Work out the finished part from the listing and answer in its coordinate system (mm). A direction names the side the tool comes from. Round coordinates to 2 decimals unless told otherwise and drop trailing zeros. Order: outer loops, then holes, each group sorted by start corner. A loop starts at its lowest first (then second) coordinate and runs counter-clockwise, first axis right, second up. Notation, with made-up numbers: (26.25, 23) -> (69.25, 23) arc R18 ccw to (69.25, 30) -> close; hole circle Ø8 at (18, -36). An arc over 180 degrees is marked (long way). Use a Markdown table: item, result. Add a question column.
Item 1: A cutting plane is placed at D-D, the plane y = 37. Determine the outline of the cut face in (x, z), plus the area to 3 significant figures.
Item 2: For a pull along X with two mould halves and no side action, classify faces 4 (the flat face through (-15.989, 44.684, -33.256)), 5 (the flat face through (0, 53, -38.354)), 6 (the flat face through (16.079, 99.775, -33.256)), 7 (the cylindrical face through (0.704, -3.131, 31.996)) as +X half, -X half, draft (parallel to the pull), parting line (faces both ways), or undercut.
Item 3: Flat-ended cylindrical pins translate along their axes: P1, Ø12, axis at x = -0.5, z = -21.5, coming from the +Y side; P2, Ø7, axis at y = 50.5, z = -34, coming from the +X side; P3, Ø10.5, axis at x = -18, y = 94, coming from the +Z side; P4, Ø15.5, axis at x = 0, z = 0, coming from the -Y side. Find the tip coordinate at first contact, or state that the pin passes through.
Item 4: A cutting plane is placed at C-C, the plane x = 7. Determine the outline of the cut face in (y, z), plus the area to 3 significant figures.
Item 5: A tool of negligible diameter and unlimited length cuts with its end or side. For faces 1 (the flat face through (0, -6.35, -11)), 2 (the flat face through (-29, 100.076, -35)), 3 (the flat face through (16.079, 44.736, -33.256)), from which of +Z, -Z, +X, -X, +Y, -Y can it reach the whole face along a straight path? Write none if from no direction.
Item 6: A cutting plane is placed at A-A, the plane x = 0. Determine the outline of the cut face in (y, z).
Item 7: A cutting plane is placed at B-B, the plane z = -25.4. Determine the outline of the cut face in (x, y), plus the area to 3 significant figures.
Item 8: Find the intervals of material crossed by L1, parallel to Z at x = 0, y = -1.85; L2, parallel to Z at x = 0, y = -5.3; L3, parallel to X at y = -1.2, z = -25.4, in increasing order. Write a range as [from, to].
from build123d import *

# Parameters (mm, degrees)
F0_R     = 9.8425
F0_W     = 64.008
F0_H     = 6.35
F1_DEPTH = 6.35
F2_DEPTH = 114.3
F3_D     = 5.5
F4_R     = 4.28625
F5_DEPTH = 2.54
F6_DEPTH = 6.351
F4_W     = 5.08
F4_H     = 14.224
F4_H_2   = 42.799
F7_DEPTH = 6.351
F9_D     = 9
F9_DEPTH = 2.54
F9_TIP   = 2.7038727856


with BuildPart() as f1:
    # F0 (on Front) → F1 (new body)
    with BuildSketch(Plane.XZ):
        with BuildLine():
            Line((32.004, -32.004), (32.004, 0))
            ThreePointArc((32.004, 0), (0, 32.004), (-32.004, 0))
            Line((-32.004, 0), (-32.004, -32.004))
            Line((-32.004, -32.004), (32.004, -32.004))
        make_face()
        Circle(F0_R, mode=Mode.SUBTRACT)
        with Locations((0, -35.179)):
            Rectangle(F0_W, F0_H)
    extrude(amount=F1_DEPTH)

    # F0 (on Front) → F2 (join)
    with BuildSketch(Plane.XZ):
        with Locations((0, -35.179)):
            Rectangle(F0_W, F0_H)
    extrude(amount=-F2_DEPTH)

    # F3 (through all)
    with Locations(Plane(origin=(0, 0, 0), x_dir=(1, 0, 0), z_dir=(0, 1, 0))):
        with Locations((0, -25.4), (0, 25.4)):
            Hole(F3_D / 2)

    # F4 (on face) → F5 (cut)
    with BuildSketch(Plane.XY.offset(-32.004)):
        Polygon((-12.827, 90.4914921457), (-12.827, 97.8971640486), (-19.2405, 101.6), (-25.654, 97.8971640486), (-25.654, 90.4914921457), (-19.2405, 86.7886561942), align=None)
        with Locations((-19.2405, 94.1943280971)):
            Circle(F4_R, mode=Mode.SUBTRACT)
        Polygon((25.654, 90.4914921457), (25.654, 97.8971640486), (19.2405, 101.6), (12.827, 97.8971640486), (12.827, 90.4914921457), (19.2405, 86.7886561942), align=None)
        with Locations((19.2405, 94.1943280971)):
            Circle(F4_R, mode=Mode.SUBTRACT)
        Polygon((25.654, 35.4528359514), (25.654, 42.8585078543), (19.2405, 46.5613438058), (12.827, 42.8585078543), (12.827, 35.4528359514), (19.2405, 31.75), align=None)
        with Locations((19.2405, 39.1556719029)):
            Circle(F4_R, mode=Mode.SUBTRACT)
        Polygon((-12.827, 35.4528359514), (-12.827, 42.8585078543), (-19.2405, 46.5613438058), (-25.654, 42.8585078543), (-25.654, 35.4528359514), (-19.2405, 31.75), align=None)
        with Locations((-19.2405, 39.1556719029)):
            Circle(F4_R, mode=Mode.SUBTRACT)
    extrude(amount=-F5_DEPTH, mode=Mode.SUBTRACT)

    # F6 (cut, through all): faces of the model
    f6_faces = [f1.faces().sort_by_distance(p)[0] for p in [
        (-19.2405, 94.1943280971, -32.004),
        (19.2405, 94.1943280971, -32.004),
        (19.2405, 39.1556719029, -32.004),
        (-19.2405, 39.1556719029, -32.004),
    ]]
    extrude(f6_faces, amount=-F6_DEPTH, mode=Mode.SUBTRACT)

    # F4 (on face) → F7 (cut, through all)
    with BuildSketch(Plane.XY.offset(-32.004)):
        with Locations((29.464, 107.188)):
            Rectangle(F4_W, F4_H)
        with Locations((29.464, 49.9745)):
            Rectangle(F4_W, F4_H_2)
        with Locations((-29.464, 107.188)):
            Rectangle(F4_W, F4_H)
        with Locations((-29.464, 49.9745)):
            Rectangle(F4_W, F4_H_2)
    extrude(amount=-F7_DEPTH, mode=Mode.SUBTRACT)

    # F9
    with Locations(Plane.XZ.offset(6.35)):
        with Locations((0, 25.4), (0, -25.4)):
            Hole(F9_D / 2, depth=F9_DEPTH)
            with Locations((0, 0, -(F9_DEPTH + F9_TIP / 2))):  # 118° drill point
                Cone(0, F9_D / 2, F9_TIP, mode=Mode.SUBTRACT)


solid = f1.part
Reported:
| question | item | result |
|---|---|---|
| 1 | outline | (-26.92, -38.35) -> (-22.95, -38.35) -> (-22.95, -34.54) -> (-25.65, -34.54) -> (-25.65, -32) -> (-26.92, -32) -> close; (-15.54, -38.35) -> (15.54, -38.35) -> (15.54, -34.54) -> (12.83, -34.54) -> (12.83, -32) -> (-12.83, -32) -> (-12.83, -34.54) -> (-15.54, -34.54) -> close; (22.95, -38.35) -> (26.92, -38.35) -> (26.92, -32) -> (25.65, -32) -> (25.65, -34.54) -> (22.95, -34.54) -> close |
| 1 | area | 220 mm² |
| 2 | face 4 | undercut |
| 2 | face 5 | draft |
| 2 | face 6 | undercut |
| 2 | face 7 | parting line |
| 3 | P1 | y = 0 |
| 3 | P2 | x = 26.92 |
| 3 | P3 | z = -32 |
| 3 | P4 | through |
| 4 | outline | (-6.35, -38.35) -> (114.3, -38.35) -> (114.3, -32) -> (0, -32) -> (0, -6.92) -> (-6.35, -6.92) -> close; (-6.35, 6.92) -> (0, 6.92) -> (0, 31.23) -> (-6.35, 31.23) -> close |
| 4 | area | 1,080 mm² |
| 5 | face 1 | +Z, -Z, +X, -X, -Y |
| 5 | face 2 | +Z, -Z, -X, +Y |
| 5 | face 3 | +Z |
| 6 | outline | (-6.35, -38.35) -> (114.3, -38.35) -> (114.3, -32) -> (0, -32) -> (0, -28.15) -> (-2.76, -28.15) -> (-3.81, -29.9) -> (-6.35, -29.9) -> close; (-6.35, -20.9) -> (-3.81, -20.9) -> (-2.76, -22.65) -> (0, -22.65) -> (0, -9.84) -> (-6.35, -9.84) -> close; (-6.35, 9.84) -> (0, 9.84) -> (0, 22.65) -> (-2.76, 22.65) -> (-3.81, 20.9) -> (-6.35, 20.9) -> close; (-6.35, 29.9) -> (-3.81, 29.9) -> (-2.76, 28.15) -> (0, 28.15) -> (0, 32) -> (-6.35, 32) -> close |
| 7 | outline | (-32, -6.35) -> (-4.5, -6.35) -> (-4.5, -3.81) -> (-2.75, -2.76) -> (-2.75, 0) -> (-32, 0) -> close; (2.75, -2.76) -> (4.5, -3.81) -> (4.5, -6.35) -> (32, -6.35) -> (32, 0) -> (2.75, 0) -> close |
| 7 | area | 361 mm² |
| 8 | L1 | [-38.35, -28.15], [-22.65, -9.84], [9.84, 22.65], [28.15, 32] |
| 8 | L2 | [-38.35, -29.9], [-20.9, -9.84], [9.84, 20.9], [29.9, 32] |
| 8 | L3 | [-32, -2.75], [2.75, 32] |
